Autodesk Fusion 360 part; units mm, degrees
sketch "Sketch1" plane through (0, 0, 0) normal (0, 0, 1) x (1, 0, 0)
box "BoxPrimitive1" add length 80 width 80 height 50 placed x (0, 1, 0) y (-1, 0, 0) z (0, 0, 1) at (72, 0, 0)
sketch "Sketch3" plane through (0, 0, 50) normal (0, 0, 1) x (-1, 0, 0)
  line L0 (-72, -80) -> (8, -80)
  line L1 (8, -80) -> (8, 0)
  line L2 (8, 0) -> (-72, 0)
  line L3 (-72, 0) -> (-72, -80)
  line L4 (8, 0) -> (-72, 0)
  line L5 (-72, 0) -> (-72, -80)
  line L6 (-72, -80) -> (8, -80)
  line L7 (8, -80) -> (8, 0)
  line L8 (8, 0) -> (-72, -80) construction
  line L9 (-72, 0) -> (8, -80) construction
  line L10 (6, -78) -> (-70, -78)
  line L11 (-70, -78) -> (-70, -2)
  line L12 (-70, -2) -> (6, -2)
  line L13 (6, -2) -> (6, -78)
  line L14 (6, -78) -> (-70, -2) construction
  line L15 (-70, -78) -> (6, -2) construction
  line L16 (-32, 0) -> (-32, -80)
  line L17 (8, -40) -> (-72, -40)
  point P0 (-32, -40)
  point P1 (-32, -40)
  dimension "d14" = 80
  dimension "d17" = 76
extrude "Extrude1" cut sketch "Sketch3" against normal blind 48 contours L10 L13 L16 L17 | L10 L11 L16 L17 | L11 L12 L16 L17 | L12 L13 L16 L17
sketch "Sketch4" plane through (0, 0, 0) normal (1, 0, 0) x (0, 1, 0)
  line L0 (0, 50) -> (80, 50)
  line L1 (43, 48) -> (37, 48)
  line L2 (37, 48) -> (37, 50)
  line L3 (43, 50) -> (43, 48)
  line L4 (43, 48) -> (40, 50) construction
  line L5 (37, 48) -> (40, 50) construction
extrude "Extrude2" cut sketch "Sketch4" against normal blind 10
fillet "Fillet1" radius 5 4 edges at (-6, 78, 26) (-6, 2, 26) (70, 2, 26) (70, 78, 26)
sketch "Sketch6" plane through (0, 0, 0) normal (0, -1, 0) x (1, 0, 0)
  line L0 (-8, 50) -> (-8, 0)
  line L1 (-8, 0) -> (72, 0)
  line L2 (72, 0) -> (72, 50)
  line L3 (72, 50) -> (-8, 50)
ref_plane "WorkPlane1" through (0, 40, 0) normal (0, -1, 0) x (1, 0, 0)
sketch "Sketch7" plane through (0, 40, 0) normal (0, -1, 0) x (-1, 0, 0)
fillet "Fillet2" radius 0.5 2 edges at (-7, 37, 48) (-7, 43, 48)
sketch "Sketch8" plane through (0, 0, 2) normal (0, 0, 1) x (-1, 0, 0)
  circle A0 centre (-32, -40) radius 30
  circle A1 centre (-32, -40) radius 32
  line L0 (-32, -40) -> (-32, -7)
  line L1 (-32, -40) -> (-32, -72)
  line L2 (-32, -40) -> (0, -40)
  line L3 (-32, -40) -> (-64, -40)
  line L4 (-32, -40) -> (-9.3726, -62.6274)
  line L5 (-32, -40) -> (-54.6505, -62.6505)
  line L6 (-32, -40) -> (-64.0327, -40) construction
  line L7 (-32, -40) -> (-9.3726, -17.3726)
  line L8 (-32, -40) -> (0, -40) construction
  line L9 (-32, -40) -> (-54.6274, -17.3726)
  line L10 (-32, -40) -> (-64, -40) construction
  arc A2 (-70, -73) -> (-65, -78) centre (-65, -73) ccw
  line L11 (-65, -78) -> (1, -78)
  arc A3 (1, -78) -> (6, -73) centre (1, -73) ccw
  line L12 (6, -73) -> (6, -7)
  arc A4 (6, -7) -> (1, -2) centre (1, -7) ccw
  line L13 (1, -2) -> (-65, -2)
  arc A5 (-65, -2) -> (-70, -7) centre (-65, -7) ccw
  line L14 (-70, -7) -> (-70, -73)
  dimension "d29" = 45
  dimension "d30" = 45
  dimension "d31" = 45
  dimension "d32" = 45
extrude "Extrude3" add sketch "Sketch8" along normal blind 5 contours A0 A1 L0 L7 | A0 A1 L1 L4 | A0 A1 L0 L9 | A0 A1 L1 L5
fillet "Fillet3" radius 5 4 edges at (72, 80, 25) (72, 0, 25) (-8, 80, 25) (-8, 0, 25)
The listing builds one solid part. Answer for the finished solid, in the listing's coordinates (mm). A direction names the side the tool comes from. Give positions to 0.01 mm unless a question says otherwise; leave off trailing zeros. Order: outer loops, then holes, each group sorted by start corner. A loop starts at its lowest first (then second) coordinate and runs counter-clockwise, first axis right, second up.
1) Given P1, Ø8, axis at x = 19, y = 57.5, coming from the +Z side; P2, Ø0.8, axis at x = -7.5, z = 49.5, coming from the -Y side; P3, Ø2, axis at x = -7.5, y = 40, coming from the +Z side, each flat-ended and moving along its own axis, determine where each tip first touches the part or whether it passes through.
Reported:
P1: stops at z = 2
P2: stops at y = 2.14
P3: stops at z = 48
2) Determine the mould class of faces 1 (the face through (32, 0, 25)), 2 (the face through (32, 80, 25)), 3 (the face through (69, 4, 26)), 4 (the face through (72, 40, 25)) for opening direction Y: pulls with the +Y half, pulls with the -Y half, needs draft (parallel to the pull), parting line crosses it, or undercut.
Reported:
face 1: pulls with the -Y half
face 2: pulls with the +Y half
face 3: undercut
face 4: needs draft
3) For faces 5 (the face through (32, 78, 26)), 6 (the face through (-6, 79, 25)), 7 (the face through (-7, 40, 48)), determine the directions among +Z, -Z, +X, -X, +Y, -Y from which every point of the face is accessible in a straight line to the end or side of a thin tool.
Reported:
face 5: +Z
face 6: +Z, -Z, -X, +Y
face 7: +Z, -X
4) Consider line 1 along X through (y, z) = (62.5, 19); line 2 along Y through (x, z) = (51, 4.5); line 3 along Y through (x, z) = (27, 16.5). Determine where each line is inside the solid, lowest interval first.
Reported:
line 1: x = -8 to -6, 70 to 72
line 2: y = 0 to 2, 14.25 to 16.78, 63.22 to 65.75, 78 to 80
line 3: y = 0 to 2, 78 to 80
5) Find section B-B on y = 35. Write down the section's boundary in (x, z).
Reported:
outline: (-8, 0) - (72, 0) - (72, 50) - (70, 50) - (70, 2) - (-6, 2) - (-6, 50) - (-8, 50) - close
6) Find section C-C on x = 7. Write down the section's boundary in (y, z), then the cut area to 3 significant figures.
Reported:
outline: (0, 0) - (80, 0) - (80, 50) - (78, 50) - (78, 2) - (2, 2) - (2, 50) - (0, 50) - close
area: 352 mm2
7) Find section D-D on x = 39. Write down the section's boundary in (y, z).
Reported:
outline: (0, 0) - (80, 0) - (80, 50) - (78, 50) - (78, 2) - (71.22, 2) - (71.22, 7) - (69.17, 7) - (69.17, 2) - (10.83, 2) - (10.83, 7) - (8.78, 7) - (8.78, 2) - (2, 2) - (2, 50) - (0, 50) - close
8) Find section A-A on z = 34.5. Write down the section's boundary in (x, y), then the cut area to 3 significant figures.
Reported:
outline: (-8, 5) arc R5 ccw to (-3, 0) - (67, 0) arc R5 ccw to (72, 5) - (72, 75) arc R5 ccw to (67, 80) - (-3, 80) arc R5 ccw to (-8, 75) - close; hole (-6, 7) arc R5 ccw to (-1, 2) - (65, 2) arc R5 ccw to (70, 7) - (70, 73) arc R5 ccw to (65, 78) - (-1, 78) arc R5 ccw to (-6, 73) - close
area: 624 mm2
